from build123d import *

# Parameters (mm, degrees)
SKETCH1_W               = 116.5
SKETCH1_H               = 15
BOSS_EXTRUDE1_DEPTH     = 1
SKETCH2_W               = 20
SKETCH2_H               = 15
BOSS_EXTRUDE2_DEPTH     = 4
CUT_EXTRUDE1_DEPTH      = 97.920070161
MIRROR2_COPY_1_SKETCH_W = 20
MIRROR2_COPY_1_SKETCH_H = 15
MIRROR2_COPY_1_DEPTH    = 4
MIRROR2_COPY_2_DEPTH    = 97.920070161
BOSS_EXTRUDE5_DEPTH     = 1.5
CUT_EXTRUDE2_DEPTH      = 60.783463433
SKETCH9_R               = 0.75
CUT_EXTRUDE3_DEPTH      = 117.954050806


with BuildPart() as part:
    # Sketch1 → Boss-Extrude1 (new, symmetric)
    with BuildSketch(Plane(origin=(0, 0, 0), x_dir=(0, 0, -1), z_dir=(1, 0, 0))):
        Rectangle(SKETCH1_W, SKETCH1_H)
    extrude(amount=BOSS_EXTRUDE1_DEPTH, both=True)

    # Sketch2 → Boss-Extrude2 (add)
    with BuildSketch(Plane(origin=(1, 0, 0), x_dir=(0, 0, -1), z_dir=(1, 0, 0))):
        with Locations((48.25, 0)):
            Rectangle(SKETCH2_W, SKETCH2_H)
    boss_extrude2 = extrude(amount=BOSS_EXTRUDE2_DEPTH)

    # Sketch3 → Cut-Extrude1 (cut, through all)
    with BuildSketch(Plane.XY.offset(-38.25)):
        Polygon((5, 2.5), (1, 5), (1, -5), (5, -2.5), align=None)
    cut_extrude1 = extrude(amount=-CUT_EXTRUDE1_DEPTH, mode=Mode.SUBTRACT)

    # Mirror1: Boss-Extrude2, Cut-Extrude1 across plane
    add(boss_extrude2.mirror(Plane(origin=(0, 0, 0), x_dir=(0, 0, 1), z_dir=(1, 0, 0))))
    add(cut_extrude1.mirror(Plane(origin=(0, 0, 0), x_dir=(0, 0, 1), z_dir=(1, 0, 0))), mode=Mode.SUBTRACT)

    # Mirror2: Boss-Extrude2, Cut-Extrude1 across plane
    add(boss_extrude2.mirror(Plane.XY))
    add(cut_extrude1.mirror(Plane.XY), mode=Mode.SUBTRACT)

    # Mirror2 copy 1 sketch → Mirror2 copy 1 (add)
    with BuildSketch(Plane.ZY.offset(1)):
        with Locations((48.25, 0)):
            Rectangle(MIRROR2_COPY_1_SKETCH_W, MIRROR2_COPY_1_SKETCH_H)
    extrude(amount=MIRROR2_COPY_1_DEPTH)

    # Mirror2 copy 2 sketch → Mirror2 copy 2 (cut, through all)
    with BuildSketch(Plane(origin=(0, 0, 38.25), x_dir=(-1, 0, 0), z_dir=(0, 0, -1))):
        Polygon((5, 2.5), (1, 5), (1, -5), (5, -2.5), align=None)
    extrude(amount=-MIRROR2_COPY_2_DEPTH, mode=Mode.SUBTRACT)

    # Sketch7 → Boss-Extrude5 (add)
    with BuildSketch(Plane(origin=(0, 7.5, 0), x_dir=(1, 0, 0), z_dir=(0, 1, 0))):
        Polygon((0, -58.25), (-5, -38.25), (-5, 38.25), (0, 58.25), (5, 38.25), (5, -38.25), align=None)
    boss_extrude5 = extrude(amount=BOSS_EXTRUDE5_DEPTH)

    # Sketch8 → Cut-Extrude2 (cut, through all)
    with BuildSketch(Plane.ZY.offset(5)):
        Polygon((-38.25, 9), (-58.25, 7.5), (-58.25, 9), align=None)
        Polygon((58.25, 9), (38.25, 9), (58.25, 7.5), align=None)
    cut_extrude2 = extrude(amount=-CUT_EXTRUDE2_DEPTH, mode=Mode.SUBTRACT)

    # Sketch9 → Cut-Extrude3 (cut, through all)
    with BuildSketch(Plane.XY.offset(58.25)):
        with Locations((1.2, 8.7)):
            Circle(SKETCH9_R)
        with Locations((-1.2, 8.7)):
            Circle(SKETCH9_R)
    cut_extrude3 = extrude(amount=-CUT_EXTRUDE3_DEPTH, mode=Mode.SUBTRACT)

    # Mirror4: Boss-Extrude5, Cut-Extrude2, Cut-Extrude3 across plane
    add(boss_extrude5.mirror(Plane.ZX))
    add(cut_extrude2.mirror(Plane.ZX), mode=Mode.SUBTRACT)
    add(cut_extrude3.mirror(Plane.ZX), mode=Mode.SUBTRACT)


solid = part.part
Design review of the part built by this model. Coordinates are the model's own, in mm. A direction names the side the tool comes from. Give positions to 0.01 mm unless a question says otherwise; leave off trailing zeros. Write each loop counter-clockwise with the first axis right and the second up, starting at its lowest first coordinate (ties: lowest second). Pieces come first, ordered by that corner, then holes. Notation, with made-up numbers: M 68.5,32 L 91.5,32 A19 cw 91.5,41 Z; hole C 3,26.25 d9. An arc over 180 degrees is marked long. Return JSON: item names as keys, results as strings. Group by question number.
Item 1: Take a section at A-A (y = 4). Give the boundary of the cut face in (x, z).
Item 2: The part is to be moulded in two halves that separate along X. For faces 1 (the flat face through (-5, 5, 48)), 2 (the flat face through (3.03, 3.73, 48.11)), 3 (the flat face through (2.97, -3.77, 48.11)), 4 (the flat face through (-4, -7.5, 53)), say which applies: pulls with the +X half, pulls with the -X half, needs draft (parallel to the pull), parting line crosses it, or undercut.
Item 3: Take a section at B-B (x = -3.25). Give the boundary of the cut face in (y, z) (3 decimals).
Item 4: Wall thickness on line 1 along X through (y, z) = (8.7, -29); line 2 along Y through (x, z) = (1.2, 18.5); line 3 along Y through (x, z) = (4.25, -24): over which ranges is each line inside the solid? List them lowest first.
Item 5: Take a section at D-D (y = -0.75). Give the boundary of the cut face in (x, z), plus the area to 3 significant figures.
Item 6: Take a section at C-C (z = 30). Give the boundary of the cut face in (x, y), plus the area to 3 significant figures.
Item 7: Clearance check with flat-ended pins moving along their axes: pin 1 Ø3 at (y, z) = (2, -29.5) entering from -X; pin 2 Ø2 at (y, z) = (-0.5, -9.5) entering from +X; pin 3 Ø1.5 at (x, z) = (2, 45.5) entering from +Y; pin 4 Ø1.4 at (x, y) = (-1.2, 8.7) entering from -Z. State where each tip first meets the part, or that it passes through.
Item 8: Tool access review of faces 5 (the flat face through (3, 7.5, -1)), 6 (the flat face through (3.09, 8.07, 45.89)), 7 (the flat face through (2.97, -3.77, -48.11)), 8 (the flat face through (1, 0, 1)): name each direction out of +Z, -Z, +X, -X, +Y, -Y from which nothing blocks a thin tool from reaching the whole face with its end or side.
Return value:
{
 "1": {"outline": "M -5,-58.25 L -2.6,-58.25 L -2.6,-38.25 L -5,-38.25 Z; M -5,38.25 L -2.6,38.25 L -2.6,58.25 L -5,58.25 Z; M -1,-58.25 L 1,-58.25 L 1,58.25 L -1,58.25 Z; M 2.6,-58.25 L 5,-58.25 L 5,-38.25 L 2.6,-38.25 Z; M 2.6,38.25 L 5,38.25 L 5,58.25 L 2.6,58.25 Z"},
 "2": {"face 1": "pulls with the -X half", "face 2": "undercut", "face 3": "undercut", "face 4": "needs draft"},
 "3": {"outline": "M -9,-38.25 L -8.475,-45.25 L -7.5,-45.25 L -7.5,-58.25 L -3.594,-58.25 L -3.594,-38.25 L -7.5,-38.25 L -7.5,38.25 L -3.594,38.25 L -3.594,58.25 L -7.5,58.25 L -7.5,45.25 L -8.475,45.25 L -9,38.25 Z; M 3.594,-58.25 L 7.5,-58.25 L 7.5,-45.25 L 8.475,-45.25 L 9,-38.25 L 9,38.25 L 8.475,45.25 L 7.5,45.25 L 7.5,58.25 L 3.594,58.25 L 3.594,38.25 L 7.5,38.25 L 7.5,-38.25 L 3.594,-38.25 Z"},
 "4": {"line 1": "x = -5 to -1.95, -0.45 to 0.45, 1.95 to 5", "line 2": "y = -7.95 to -7.5, 7.5 to 7.95", "line 3": "y = -9 to -7.5, 7.5 to 9"},
 "5": {"outline": "M -1,-58.25 L 1,-58.25 L 1,58.25 L -1,58.25 Z", "area": "233 mm2"},
 "6": {"outline": "M -5,-9 L -1.89,-9 A0.75 cw long -0.51,-9 L 0.51,-9 A0.75 cw long 1.89,-9 L 5,-9 L 5,-7.5 L 1,-7.5 L 1,7.5 L 5,7.5 L 5,9 L 1.89,9 A0.75 cw long 0.51,9 L -0.51,9 A0.75 cw long -1.89,9 L -5,9 L -5,7.5 L -1,7.5 L -1,-7.5 L -5,-7.5 Z", "area": "54.7 mm2"},
 "7": {"pin 1": "stops at x = -1", "pin 2": "stops at x = 1", "pin 3": "stops at y = 8.51", "pin 4": "passes through"},
 "8": {"face 5": "+X", "face 6": "+Z, +X, +Y", "face 7": "+Z, -Z", "face 8": "none"}
}
